Design review of the part built by this model. Coordinates are the model's own, in mm. A direction names the side the tool comes from. Coordinates: 2 decimals unless noted, no trailing zeros. Order: outer loops, then holes, each group sorted by start corner. A loop starts at its lowest first (then second) coordinate and runs counter-clockwise, first axis right, second up. Notation, with made-up numbers: M -35,59.25 L 10,59.25 A32 ccw 10,90.25 Z; hole C 37.5,-29.5 d5. An arc over 180 degrees is marked long. Answer in a Markdown table with one row per item.
from build123d import *

# Parameters (mm, degrees)
SKETCH1_R              = 32
BOSS_EXTRUDE1_DEPTH    = 15
FILLET1_R              = 10
SHELL1_T               = -2
SKETCH2_W              = 15
SKETCH2_H              = 10
BOSS_EXTRUDE2_DEPTH    = 5
SKETCH3_R              = 29
CUT_EXTRUDE1_DEPTH     = 5
SPLIT1_SURFACE_1_BACK  = 146
SPLIT1_SURFACE_1_DEPTH = 292
SPLIT1_SURFACE_2_BACK  = 146
SPLIT1_SURFACE_2_DEPTH = 292
SKETCH6_R              = 2.5
SKETCH6_R_2            = 1
BOSS_EXTRUDE3_DEPTH    = 5
BOSS_EXTRUDE4_START    = 5
SKETCH5_R              = 2.5
SKETCH5_R_2            = 1
BOSS_EXTRUDE4_DEPTH    = 5
SKETCH7_W              = 8.5
SKETCH7_H              = 13.5
BOSS_EXTRUDE5_DEPTH    = 5.5
SKETCH8_W              = 8.5
SKETCH8_H              = 13.5
BOSS_EXTRUDE6_DEPTH    = 5.5
FILLET3_R              = 1
FILLET4_R              = 10
SKETCH9_W              = 1
SKETCH9_H              = 5.049910015
SKETCH9_H_2            = 5
CUT_EXTRUDE2_DEPTH     = 10


with BuildPart() as part:
    # Sketch1 → Boss-Extrude1 (new body)
    with BuildSketch(Plane.XY):
        Circle(SKETCH1_R)
    extrude(amount=BOSS_EXTRUDE1_DEPTH)

    # Fillet1
    fillet1_edges = [part.edges().sort_by_distance(p)[0] for p in [
        (-32, 0, 15),
    ]]
    fillet(fillet1_edges, radius=FILLET1_R)

    # Shell1
    shell1_openings = [part.faces().sort_by_distance(p)[0] for p in [
        (0, 0, 0),
    ]]
    offset(amount=SHELL1_T, openings=shell1_openings, kind=Kind.INTERSECTION)

    # Sketch2 → Boss-Extrude2 (add)
    with BuildSketch(Plane(origin=(0, 0, 0), x_dir=(-1, 0, 0), z_dir=(0, 0, -1))):
        with BuildLine():
            Line((-60, 10), (-38.729833462, 10))
            ThreePointArc((-38.729833462, 10), (0, 40), (38.729833462, 10))
            Line((38.729833462, 10), (60, 10))
            Line((60, 10), (60, -10))
            Line((60, -10), (38.729833462, -10))
            ThreePointArc((38.729833462, -10), (0, -40), (-38.729833462, -10))
            Line((-38.729833462, -10), (-60, -10))
            Line((-60, -10), (-60, 10))
        make_face()
        with Locations((-47.5, 0.049910015)):
            Rectangle(SKETCH2_W, SKETCH2_H, mode=Mode.SUBTRACT)
        with Locations((47.5, 0)):
            Rectangle(SKETCH2_W, SKETCH2_H, mode=Mode.SUBTRACT)
    extrude(amount=-BOSS_EXTRUDE2_DEPTH)

    # Sketch3 → Cut-Extrude1 (cut)
    with BuildSketch(Plane(origin=(0, 0, 0), x_dir=(-1, 0, 0), z_dir=(0, 0, -1))):
        Circle(SKETCH3_R)
    extrude(amount=-CUT_EXTRUDE1_DEPTH, mode=Mode.SUBTRACT)


with BuildPart() as body_2:
    # Split1: the piece behind the surface
    add(part.part)
    # Split1 surface: a surface, the sketch's curves swept straight by 292 mm
    with BuildLine(Plane(origin=(0, 0, 0), x_dir=(-1, 0, 0), z_dir=(0, 0, -1)).offset(-SPLIT1_SURFACE_1_BACK), mode=Mode.PRIVATE) as split1_surface_1_path:
        Line((-60, 0), (60, 0))
    split1_surface_1 = Shell.extrude(split1_surface_1_path.wire(), (0 * SPLIT1_SURFACE_1_DEPTH, 0 * SPLIT1_SURFACE_1_DEPTH, -1 * SPLIT1_SURFACE_1_DEPTH))
    split(bisect_by=split1_surface_1, keep=Keep.BOTTOM)


with BuildPart() as part_1:
    add(part.part)

    # Split1: split by a surface, the side it looks to stays
    # Split1 surface: a surface, the sketch's curves swept straight by 292 mm
    with BuildLine(Plane(origin=(0, 0, 0), x_dir=(-1, 0, 0), z_dir=(0, 0, -1)).offset(-SPLIT1_SURFACE_2_BACK), mode=Mode.PRIVATE) as split1_surface_2_path:
        Line((-60, 0), (60, 0))
    split1_surface_2 = Shell.extrude(split1_surface_2_path.wire(), (0 * SPLIT1_SURFACE_2_DEPTH, 0 * SPLIT1_SURFACE_2_DEPTH, -1 * SPLIT1_SURFACE_2_DEPTH))
    split(bisect_by=split1_surface_2, keep=Keep.TOP)

    # Sketch6 → Boss-Extrude3 (add)
    with BuildSketch(Plane.ZY.offset(-55)):
        Circle(SKETCH6_R)
        Circle(SKETCH6_R_2, mode=Mode.SUBTRACT)
    extrude(amount=BOSS_EXTRUDE3_DEPTH)

    # Sketch5 → Boss-Extrude4 (add)
    with BuildSketch(Plane(origin=(-55, 0, 0), x_dir=(0, 0, -1), z_dir=(1, 0, 0)).offset(BOSS_EXTRUDE4_START)):
        with Locations(Location((0, 0, 0), (0, 0, 180))):
            Circle(SKETCH5_R)
        with Locations(Location((0, 0, 0), (0, 0, 180))):
            Circle(SKETCH5_R_2, mode=Mode.SUBTRACT)
    extrude(amount=-BOSS_EXTRUDE4_DEPTH)

    # Sketch7 → Boss-Extrude5 (add)
    with BuildSketch(Plane(origin=(60, 0, 0), x_dir=(0, 0, -1), z_dir=(1, 0, 0))):
        with Locations((-0.75, 3.25)):
            Rectangle(SKETCH7_W, SKETCH7_H)
    extrude(amount=-BOSS_EXTRUDE5_DEPTH)

    # Sketch8 → Boss-Extrude6 (add)
    with BuildSketch(Plane.ZY.offset(60)):
        with Locations((0.75, 3.25)):
            Rectangle(SKETCH8_W, SKETCH8_H)
    extrude(amount=-BOSS_EXTRUDE6_DEPTH)

    # Fillet3
    fillet3_edges = [part_1.edges().sort_by_distance(p)[0] for p in [
        (60, 3.25, 5),
        (-60, 3.25, 5),
        (-60, 10, 0.75),
        (60, 10, 0.75),
        (54.5, 5.049910015, 2.5),
        (54.5, 7.524955008, 0),
        (54.5, 0, -2.5),
        (60, 3.25, -3.5),
        (60, -3.5, 0.75),
        (-54.5, 0, -2.5),
        (-54.5, 7.5, 0),
        (-54.5, 5, 2.5),
        (-60, -3.5, 0.75),
        (-60, 3.25, -3.5),
    ]]
    fillet(fillet3_edges, radius=FILLET3_R - 0.0001)  # a hair under: the kernel refuses the full size

    # Fillet4
    fillet4_edges = [part_1.edges().sort_by_distance(p)[0] for p in [
        (-38.729833462, 10, 2.5),
        (38.729833462, 10, 2.5),
    ]]
    fillet(fillet4_edges, radius=FILLET4_R)

    # Sketch9 → Cut-Extrude2 (cut)
    with BuildSketch(Plane(origin=(0, 0, 0), x_dir=(-1, 0, 0), z_dir=(0, 0, -1))):
        with Locations((-39.5, 2.524955008)):
            Rectangle(SKETCH9_W, SKETCH9_H)
        with Locations((39.5, 2.5)):
            Rectangle(SKETCH9_W, SKETCH9_H_2)
    extrude(amount=-CUT_EXTRUDE2_DEPTH, mode=Mode.SUBTRACT)


solid = part_1.part
(1) Add section C-C, the plane y = 33.5. Give the boundary of the cut face in (x, z).
Return value:
| item | result |
|---|---|
| outline | M -21.86,0 L 21.86,0 L 21.86,5 L -21.86,5 Z |
(2) Add section B-B, the plane x = -48. Give the boundary of the cut face in (y, z).
Return value:
| item | result |
|---|---|
| outline | M 5,0 L 10,0 L 10,5 L 5,5 Z |
(3) Draft analysis for pull direction Z (two halves, no side actions). For faces 1 (the flat face through (-57, 3, -3.5)), 2 (the flat face through (50, -1, 1)), 3 (the flat face through (-0.1, 29.5, 5)), 4 (the cylindrical face through (52, -1, 0)), state which applies: pulls with the +Z half, pulls with the -Z half, needs draft (parallel to the pull), parting line crosses it, or undercut.
Return value:
| item | result |
|---|---|
| face 1 | pulls with the -Z half |
| face 2 | needs draft |
| face 3 | undercut |
| face 4 | undercut |
(4) For line 1 along Z through (x, y) = (52.95, 0); line 2 along X through (y, z) = (4, 3.5); line 3 along X through (y, z) = (1, -0.5), list the stretches that pass through material, from the lowest coordinate up. Write a range as from..to.
Return value:
| item | result |
|---|---|
| line 1 | z = -2.5..-1, 1..2.5 |
| line 2 | x = -60..-54.5, -39..-28.72, 28.72..39, 54.5..60 |
| line 3 | x = -60..-50, 50..60 |
(5) For faces 5 (the flat face through (-9, 31, 5)), 6 (the flat face through (54, 10, 2)), 7 (the cylindrical face through (-51.7, -0.1, -2.5)), 8 (the flat face through (-39, 2, 2)), list the 3-axis set-ups (+Z, -Z, +X, -X, +Y, -Y) from which the entire face can be reached by the end or side of a thin tool; tool diameter is ignored.
Return value:
| item | result |
|---|---|
| face 5 | +Z, +Y |
| face 6 | +Z, -Z, +X, +Y |
| face 7 | none |
| face 8 | +Z, -Z, -Y |
(6) Insertion check: pin 1 Ø6.5 at (x, y) = (2.5, 13) entering from -Z; pin 2 Ø7.5 at (x, z) = (5, 10) entering from -Y; pin 3 Ø12 at (x, y) = (-9, 22) entering from -Z; pin 4 Ø1 at (y, z) = (33, 9.5) entering from +X. Each pin has a flat end and moves straight along its axis. Give the tip position at first contact, or say it passes through.
Return value:
| item | result |
|---|---|
| pin 1 | stops at z = 13 |
| pin 2 | stops at y = 0 |
| pin 3 | stops at z = 0 |
| pin 4 | passes through |
(7) Add section A-A, the plane x = 0. Give the boundary of the cut face in (y, z), and give its area (3 significant figures).
Return value:
| item | result |
|---|---|
| outline | M 0,13 L 22,13 A8 cw 30,5 L 29,5 L 29,0 L 40,0 L 40,5 L 32,5 A10 ccw 22,15 L 0,15 Z |
| area | 127 mm2 |
